Verification items for the finished model (mm, model axes). A direction names the side the tool comes from. Coordinates: 2 decimals unless noted, no trailing zeros. Order: outer loops, then holes, each group sorted by start corner. A loop starts at its lowest first (then second) coordinate and runs counter-clockwise, first axis right, second up. Notation, with made-up numbers: M 14,-12 L 73,-12 A29 ccw 73,25 Z; hole C 16,73.5 d5. An arc over 180 degrees is marked long. Answer as a JSON object with one key per item and string values. Group by question number.
(1) Gauge pin test, flat ends, axial feed: pin 1 Ø6.5 at (x, y) = (74.5, -22) entering from +Z; pin 2 Ø6 at (x, y) = (64.5, 8.5) entering from -Z; pin 3 Ø2 at (y, z) = (-15.5, 1) entering from +X; pin 4 Ø2 at (y, z) = (-17, 9) entering from -X. Record the tip position at first contact, or that the pin passes through.
(2) Material ranges on line 1 (X direction, y = 20, z = 16); line 2 (Z direction, x = 24, y = 0.5); line 3 (Z direction, x = 11.5, y = -17.5), recorded low to high.
(3) Cross-section at C-C (z = -24). Enter the section's corners in (x, y).
(4) Cross-section at D-D (x = 30). Enter the section's corners in (y, z), plus the area to 3 significant figures.
(5) Cross-section at B-B (y = -9.5). Enter the section's corners in (x, z), plus the area to 3 significant figures.
(6) Cross-section at A-A (x = 78.5). Enter the section's corners in (y, z).
(7) Access from +Z, -Z, +X, -X, +Y, -Y to the whole of each face (thin tool, end or side, straight path). Record for faces 1 (the face through (76.2, 3, 7)), 2 (the face through (56, -22, -29.006)), 3 (the face through (56, -2.644, -23)).
from build123d import *

# Parameters (mm, degrees)
F1_DEPTH = 76.2
F2_DEPTH = 46.736
F3_DEPTH = 114.3


with BuildPart() as f1:
    # F0 (on Right) → F1 (new body)
    with BuildSketch(Plane.YZ):
        Polygon((22.755747968, 21.8976219215), (-15.344252032, 21.8976219215), (-15.344252032, -16.3060310256), (-2.644252032, -16.3060310256), (-2.644252032, -3.5023780785), (22.755747968, -3.5023780785), align=None)
        Polygon((-15.344252032, -29.0060310256), (-28.044252032, -29.0060310256), (-28.044252032, -41.7060310256), (-2.644252032, -41.7060310256), (-2.644252032, -16.3060310256), (-15.344252032, -16.3060310256), align=None)
    extrude(amount=F1_DEPTH)

    # F2 (add): a face of the model
    f2_faces = [f1.faces().sort_by_distance(p)[0] for p in [
        (0, -2.6494304529, -4.812812026),
    ]]
    extrude(f2_faces, amount=-F2_DEPTH)

    # F0 (on Right) → F3 (join)
    with BuildSketch(Plane.YZ):
        Polygon((-15.344252032, -29.0060310256), (-28.044252032, -29.0060310256), (-28.044252032, -41.7060310256), (-2.644252032, -41.7060310256), (-2.644252032, -16.3060310256), (-15.344252032, -16.3060310256), align=None)
    extrude(amount=F3_DEPTH)


solid = f1.part
Taken from the geometry:
{
 "1": {"pin 1": "stops at z = -29.01", "pin 2": "stops at z = -3.5", "pin 3": "stops at x = 76.2", "pin 4": "passes through"},
 "2": {"line 1": "x = 0 to 76.2", "line 2": "z = -3.5 to 21.9", "line 3": "z = -41.71 to -29.01"},
 "3": {"outline": "M 0,-15.34 L 114.3,-15.34 L 114.3,-2.64 L 0,-2.64 Z"},
 "4": {"outline": "M -28.04,-41.71 L -2.64,-41.71 L -2.64,-3.5 L 22.76,-3.5 L 22.76,21.9 L -15.34,21.9 L -15.34,-29.01 L -28.04,-29.01 Z", "area": "1,610 mm²"},
 "5": {"outline": "M 0,-41.71 L 114.3,-41.71 L 114.3,-16.31 L 76.2,-16.31 L 76.2,21.9 L 0,21.9 Z", "area": "5,810 mm²"},
 "6": {"outline": "M -28.04,-41.71 L -2.64,-41.71 L -2.64,-16.31 L -15.34,-16.31 L -15.34,-29.01 L -28.04,-29.01 Z"},
 "7": {"face 1": "+Z, +X, +Y, -Y", "face 2": "+Z, +X, -X, -Y", "face 3": "-Z, +X, -X, +Y"}
}
